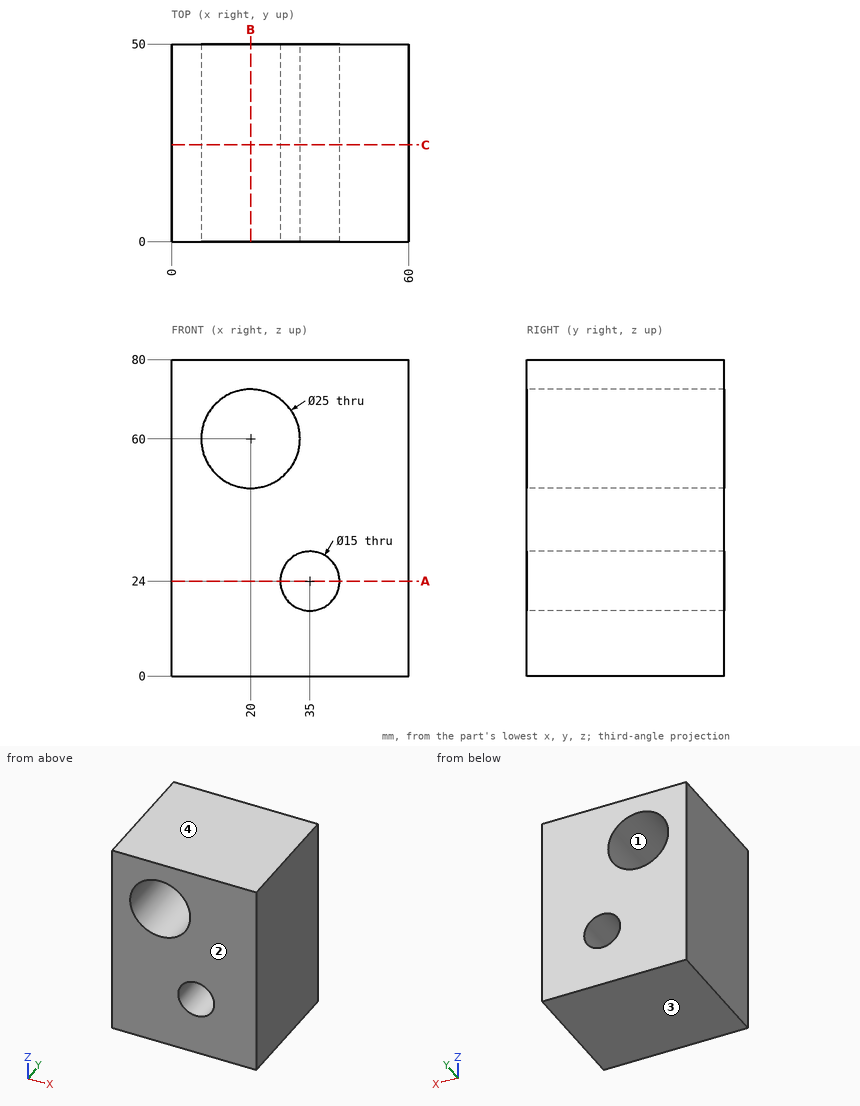
Source: three-view drawing plus pictorial views. Frame: mm from the lowest corner of the part. Round coordinates to 2 decimals unless told otherwise and drop trailing zeros. Order: outer loops, then holes, each group sorted by start corner. A loop starts at its lowest first (then second) coordinate and runs counter-clockwise, first axis right, second up. Notation, with made-up numbers: (54, 77.5) -> (63, 77.5) arc R19 cw to (63, 88.5) -> close; hole circle Ø5 at (-9, 9). An arc over 180 degrees is marked (long way). Use one line per item in the form item = value. Start each with the question number.
1. Cut plane A-A (z = 24). Return the cut outline in (x, y).
2. Cut plane C-C (y = 24.5). Return the cut outline in (x, z), then the cut area to 3 significant figures.
3. Cut plane B-B (x = 20). Return the cut outline in (y, z).
4. Draft query along Z for the marked faces 1, 2, 3 and 4. Return one class per face: pulls with the +Z half, pulls with the -Z half, needs draft (parallel to the pull), parting line crosses it, or undercut.
5. Line query: probe 1 along Z at (x, y) = (35, 27); probe 2 along Z at (x, y) = (29, 21.5); probe 3 along Z at (x, y) = (20, 14). Output: solid intervals per line, ascending.
Solution:
q1.outline = (0, 0) -> (27.5, 0) -> (27.5, 50) -> (0, 50) -> close; (42.5, 0) -> (60, 0) -> (60, 50) -> (42.5, 50) -> close
q2.outline = (0, 0) -> (60, 0) -> (60, 80) -> (0, 80) -> close; hole circle Ø25 at (20, 60); hole circle Ø15 at (35, 24)
q2.area = 4,130 mm^2
q3.outline = (0, 0) -> (50, 0) -> (50, 47.5) -> (0, 47.5) -> close; (0, 72.5) -> (50, 72.5) -> (50, 80) -> (0, 80) -> close
q4.face_1 = undercut
q4.face_2 = needs draft
q4.face_3 = pulls with the -Z half
q4.face_4 = pulls with the +Z half
q5.probe_1 = 0 to 16.5, 31.5 to 80
q5.probe_2 = 0 to 19.5, 28.5 to 51.33, 68.67 to 80
q5.probe_3 = 0 to 47.5, 72.5 to 80
